Verification items for the finished model (mm, model axes). Round coordinates to 2 decimals unless told otherwise and drop trailing zeros. Write each loop counter-clockwise with the first axis right and the second up, starting at its lowest first coordinate (ties: lowest second). Pieces come first, ordered by that corner, then holes.
from build123d import *

# Parameters (mm, degrees)
F0_W     = 98
F0_H     = 5
F0_R     = 5
F0_W_2   = 5
F0_H_2   = 68
F0_W_3   = 49
F1_DEPTH = 5


with BuildPart() as f1:
    # F0 (on Top) → F1 (new body)
    with BuildSketch(Plane.XY):
        with Locations((196, -172.5)):
            Rectangle(F0_W, F0_H)
        Polygon((147, -170), (245, -170), (245, -102), (245, -34), (245, 0), (0, 0), (0, -170), (49, -170), align=None)
        with Locations((25, -135)):
            Circle(F0_R, mode=Mode.SUBTRACT)
        with Locations((73, -135)):
            Circle(F0_R, mode=Mode.SUBTRACT)
        with Locations((121, -135)):
            Circle(F0_R, mode=Mode.SUBTRACT)
        with Locations((169, -135)):
            Circle(F0_R, mode=Mode.SUBTRACT)
        with Locations((217, -135)):
            Circle(F0_R, mode=Mode.SUBTRACT)
        with Locations((25, -80)):
            Circle(F0_R, mode=Mode.SUBTRACT)
        with Locations((73, -80)):
            Circle(F0_R, mode=Mode.SUBTRACT)
        with Locations((121, -80)):
            Circle(F0_R, mode=Mode.SUBTRACT)
        with Locations((25, -25)):
            Circle(F0_R, mode=Mode.SUBTRACT)
        with Locations((73, -25)):
            Circle(F0_R, mode=Mode.SUBTRACT)
        with Locations((121, -25)):
            Circle(F0_R, mode=Mode.SUBTRACT)
        with Locations((169, -80)):
            Circle(F0_R, mode=Mode.SUBTRACT)
        with Locations((217, -80)):
            Circle(F0_R, mode=Mode.SUBTRACT)
        with Locations((169, -25)):
            Circle(F0_R, mode=Mode.SUBTRACT)
        with Locations((217, -25)):
            Circle(F0_R, mode=Mode.SUBTRACT)
        with Locations((247.5, -68)):
            Rectangle(F0_W_2, F0_H_2)
        with Locations((24.5, -172.5)):
            Rectangle(F0_W_3, F0_H)
        with Locations((-24.5, -172.5)):
            Rectangle(F0_W_3, F0_H)
        Polygon((-49, -170), (0, -170), (0, 0), (-245, 0), (-245, -34), (-245, -102), (-245, -170), (-147, -170), align=None)
        with Locations((-215, -135)):
            Circle(F0_R, mode=Mode.SUBTRACT)
        with Locations((-167, -135)):
            Circle(F0_R, mode=Mode.SUBTRACT)
        with Locations((-119, -135)):
            Circle(F0_R, mode=Mode.SUBTRACT)
        with Locations((-71, -135)):
            Circle(F0_R, mode=Mode.SUBTRACT)
        with Locations((-23, -135)):
            Circle(F0_R, mode=Mode.SUBTRACT)
        with Locations((-215, -80)):
            Circle(F0_R, mode=Mode.SUBTRACT)
        with Locations((-167, -80)):
            Circle(F0_R, mode=Mode.SUBTRACT)
        with Locations((-215, -25)):
            Circle(F0_R, mode=Mode.SUBTRACT)
        with Locations((-167, -25)):
            Circle(F0_R, mode=Mode.SUBTRACT)
        with Locations((-119, -80)):
            Circle(F0_R, mode=Mode.SUBTRACT)
        with Locations((-71, -80)):
            Circle(F0_R, mode=Mode.SUBTRACT)
        with Locations((-23, -80)):
            Circle(F0_R, mode=Mode.SUBTRACT)
        with Locations((-119, -25)):
            Circle(F0_R, mode=Mode.SUBTRACT)
        with Locations((-71, -25)):
            Circle(F0_R, mode=Mode.SUBTRACT)
        with Locations((-23, -25)):
            Circle(F0_R, mode=Mode.SUBTRACT)
        Polygon((0, 0), (245, 0), (245, 34), (245, 102), (245, 170), (147, 170), (49, 170), (0, 170), align=None)
        with Locations((25, 30)):
            Circle(F0_R, mode=Mode.SUBTRACT)
        with Locations((73, 30)):
            Circle(F0_R, mode=Mode.SUBTRACT)
        with Locations((121, 30)):
            Circle(F0_R, mode=Mode.SUBTRACT)
        with Locations((25, 85)):
            Circle(F0_R, mode=Mode.SUBTRACT)
        with Locations((73, 85)):
            Circle(F0_R, mode=Mode.SUBTRACT)
        with Locations((121, 85)):
            Circle(F0_R, mode=Mode.SUBTRACT)
        with Locations((169, 30)):
            Circle(F0_R, mode=Mode.SUBTRACT)
        with Locations((217, 30)):
            Circle(F0_R, mode=Mode.SUBTRACT)
        with Locations((169, 85)):
            Circle(F0_R, mode=Mode.SUBTRACT)
        with Locations((217, 85)):
            Circle(F0_R, mode=Mode.SUBTRACT)
        with Locations((25, 140)):
            Circle(F0_R, mode=Mode.SUBTRACT)
        with Locations((73, 140)):
            Circle(F0_R, mode=Mode.SUBTRACT)
        with Locations((121, 140)):
            Circle(F0_R, mode=Mode.SUBTRACT)
        with Locations((169, 140)):
            Circle(F0_R, mode=Mode.SUBTRACT)
        with Locations((217, 140)):
            Circle(F0_R, mode=Mode.SUBTRACT)
        Polygon((-245, 0), (0, 0), (0, 170), (-49, 170), (-147, 170), (-245, 170), (-245, 102), (-245, 34), align=None)
        with Locations((-215, 30)):
            Circle(F0_R, mode=Mode.SUBTRACT)
        with Locations((-167, 30)):
            Circle(F0_R, mode=Mode.SUBTRACT)
        with Locations((-215, 85)):
            Circle(F0_R, mode=Mode.SUBTRACT)
        with Locations((-167, 85)):
            Circle(F0_R, mode=Mode.SUBTRACT)
        with Locations((-119, 30)):
            Circle(F0_R, mode=Mode.SUBTRACT)
        with Locations((-71, 30)):
            Circle(F0_R, mode=Mode.SUBTRACT)
        with Locations((-23, 30)):
            Circle(F0_R, mode=Mode.SUBTRACT)
        with Locations((-119, 85)):
            Circle(F0_R, mode=Mode.SUBTRACT)
        with Locations((-71, 85)):
            Circle(F0_R, mode=Mode.SUBTRACT)
        with Locations((-23, 85)):
            Circle(F0_R, mode=Mode.SUBTRACT)
        with Locations((-215, 140)):
            Circle(F0_R, mode=Mode.SUBTRACT)
        with Locations((-167, 140)):
            Circle(F0_R, mode=Mode.SUBTRACT)
        with Locations((-119, 140)):
            Circle(F0_R, mode=Mode.SUBTRACT)
        with Locations((-71, 140)):
            Circle(F0_R, mode=Mode.SUBTRACT)
        with Locations((-23, 140)):
            Circle(F0_R, mode=Mode.SUBTRACT)
        with Locations((247.5, 68)):
            Rectangle(F0_W_2, F0_H_2)
        with Locations((-196, -172.5)):
            Rectangle(F0_W, F0_H)
        with Locations((24.5, 172.5)):
            Rectangle(F0_W_3, F0_H)
        with Locations((-24.5, 172.5)):
            Rectangle(F0_W_3, F0_H)
        with Locations((-247.5, -68)):
            Rectangle(F0_W_2, F0_H_2)
        with Locations((-247.5, 68)):
            Rectangle(F0_W_2, F0_H_2)
        with Locations((196, 172.5)):
            Rectangle(F0_W, F0_H)
        with Locations((-196, 172.5)):
            Rectangle(F0_W, F0_H)
    extrude(amount=F1_DEPTH)


solid = f1.part
Q1. Release check for a two-part mould opening along X. For faces 1 (the cylindrical face through (221.77, -78.5, 2.46)), 2 (the flat face through (-3, 2, 0)) record: released by +X, released by -X, zero draft, split by the parting line, or undercut.
Recorded:
face 1: undercut
face 2: zero draft
Q2. Sectioned sample at A-A (x = -23). Enter the section's corners in (y, z).
Recorded:
outline: (-175, 0) - (-140, 0) - (-140, 5) - (-175, 5) - close; (-130, 0) - (-85, 0) - (-85, 5) - (-130, 5) - close; (-75, 0) - (-30, 0) - (-30, 5) - (-75, 5) - close; (-20, 0) - (25, 0) - (25, 5) - (-20, 5) - close; (35, 0) - (80, 0) - (80, 5) - (35, 5) - close; (90, 0) - (135, 0) - (135, 5) - (90, 5) - close; (145, 0) - (175, 0) - (175, 5) - (145, 5) - close
Q3. Material ranges on line 1 along X through (y, z) = (-115, 2.5); line 2 along Y through (x, z) = (-62, 4.8), recorded low to high.
Recorded:
line 1: x = -245 to 245
line 2: y = -170 to 170
Q4. Depth check by flat-ended pin: P1, Ø9, axis at x = -23, y = 140, coming from the -Z side; P2, Ø13, axis at x = -167, y = 140, coming from the +Z side; P3, Ø2, axis at x = -139, z = 3, coming from the -Y side; P4, Ø1.5, axis at y = 140.5, z = 2, coming from the -X side. Enter the tip coordinate at first touch or a pass-through.
Recorded:
P1: passes through
P2: stops at z = 5
P3: stops at y = -170
P4: stops at x = -245
Q5. Sectioned sample at B-B (y = -80). Give the number of separate pieces and of enclosed holes in the cut face, plus the area to 3 significant figures.
Recorded:
separate pieces: 11
enclosed holes: 0
area: 2,000 mm2
